Input: part model. Units: mm. Frame: model coordinates. A direction names the side the tool comes from. Coordinates: 2 decimals unless noted, no trailing zeros. Order: outer loops, then holes, each group sorted by start corner. A loop starts at its lowest first (then second) coordinate and runs counter-clockwise, first axis right, second up. Notation, with made-up numbers: (56.25, 69) -> (112.25, 69) arc R22 cw to (112.25, 106) -> close; hole circle Ø3 at (-1, 27). An arc over 180 degrees is marked (long way). Use CSV: the item, a comma, the result in double quotes. Start each with the question number.
```python
from build123d import *

# Parameters (mm, degrees)
BOX002_W          = 4.2
BOX002_H          = 3
BOX002_DEPTH      = 4
CYLINDER005_R     = 2.1
CYLINDER005_DEPTH = 4
CYLINDER004_R     = 2.1
CYLINDER004_DEPTH = 4
BOX003_W          = 9
BOX003_H          = 3
BOX003_DEPTH      = 4
CYLINDER006_R     = 4.5
CYLINDER006_DEPTH = 4
CYLINDER007_R     = 4.5
CYLINDER007_DEPTH = 4
BOX005_W          = 6
BOX005_H          = 8
BOX005_DEPTH      = 4
CHAMFER002_SIZE   = 2
BOX006_W          = 60
BOX006_H          = 8
BOX006_DEPTH      = 4
CHAMFER_SIZE      = 2
CHAMFER003_SIZE   = 2
BOX004_W          = 6
BOX004_H          = 8
BOX004_DEPTH      = 4
CHAMFER001_SIZE   = 2
BOX_W             = 4.2
BOX_H             = 3
BOX_DEPTH         = 4
CYLINDER001_R     = 2.1
CYLINDER001_DEPTH = 4
CYLINDER_R        = 2.1
CYLINDER_DEPTH    = 4
BOX001_W          = 9
BOX001_H          = 3
BOX001_DEPTH      = 4
CYLINDER003_R     = 4.5
CYLINDER003_DEPTH = 4
CYLINDER002_R     = 4.5
CYLINDER002_DEPTH = 4


with BuildPart() as obj1:
    # Box002 → Box002 (new body)
    with BuildSketch(Plane(origin=(-2.1, 0, 0), x_dir=(1, 0, 0), z_dir=(0, 0, 1))):
        with Locations((2.1, 1.5)):
            Rectangle(BOX002_W, BOX002_H)
    extrude(amount=BOX002_DEPTH)


with BuildPart() as zylinder005:
    # Cylinder005 → Cylinder005 (new body)
    with BuildSketch(Plane(origin=(0, 3, 0), x_dir=(1, 0, 0), z_dir=(0, 0, 1))):
        Circle(CYLINDER005_R)
    extrude(amount=CYLINDER005_DEPTH)


with BuildPart() as fusion002:
    # Cylinder004 → Cylinder004 (new body)
    with BuildSketch(Plane.XY):
        Circle(CYLINDER004_R)
    extrude(amount=CYLINDER004_DEPTH)

    # Fusion002: union obj1, Zylinder005
    add(obj1.part)
    add(zylinder005.part)


with BuildPart() as obj2:
    # Box003 → Box003 (new body)
    with BuildSketch(Plane(origin=(-4.5, 0, 0), x_dir=(1, 0, 0), z_dir=(0, 0, 1))):
        with Locations((4.5, 1.5)):
            Rectangle(BOX003_W, BOX003_H)
    extrude(amount=BOX003_DEPTH)


with BuildPart() as zylinder006:
    # Cylinder006 → Cylinder006 (new body)
    with BuildSketch(Plane(origin=(0, 3, 0), x_dir=(1, 0, 0), z_dir=(0, 0, 1))):
        Circle(CYLINDER006_R)
    extrude(amount=CYLINDER006_DEPTH)


with BuildPart() as cut001:
    # Cylinder007 → Cylinder007 (new body)
    with BuildSketch(Plane.XY):
        Circle(CYLINDER007_R)
    extrude(amount=CYLINDER007_DEPTH)

    # Fusion003: union obj2, Zylinder006
    add(obj2.part)
    add(zylinder006.part)

    # Cut001: cut Fusion002
    add(fusion002.part, mode=Mode.SUBTRACT)


with BuildPart() as cut001_1:
    # Cut001 placement: moved
    add(cut001.part.moved(Location((77.5, 0, 0))))


with BuildPart() as chamfer002:
    # Box005 → Box005 (new body)
    with BuildSketch(Plane(origin=(69, -3.5, 0), x_dir=(1, 0, 0), z_dir=(0, 0, 1))):
        with Locations((3, 4)):
            Rectangle(BOX005_W, BOX005_H)
    extrude(amount=BOX005_DEPTH)

    # Chamfer002
    chamfer002_edges = [chamfer002.edges().sort_by_distance(p)[0] for p in [
        (69, 0.5, 0),
    ]]
    chamfer(chamfer002_edges, length=CHAMFER002_SIZE)


with BuildPart() as chamfer003:
    # Box006 → Box006 (new body)
    with BuildSketch(Plane(origin=(11, -3.5, 2), x_dir=(1, 0, 0), z_dir=(0, 0, 1))):
        with Locations((30, 4)):
            Rectangle(BOX006_W, BOX006_H)
    extrude(amount=BOX006_DEPTH)

    # Chamfer
    chamfer_edges = [chamfer003.edges().sort_by_distance(p)[0] for p in [
        (11, 0.5, 6),
    ]]
    chamfer(chamfer_edges, length=CHAMFER_SIZE)

    # Chamfer003
    chamfer003_edges = [chamfer003.edges().sort_by_distance(p)[0] for p in [
        (71, 0.5, 6),
    ]]
    chamfer(chamfer003_edges, length=CHAMFER003_SIZE)


with BuildPart() as fusion004:
    # Box004 → Box004 (new body)
    with BuildSketch(Plane(origin=(7, -3.5, 0), x_dir=(1, 0, 0), z_dir=(0, 0, 1))):
        with Locations((3, 4)):
            Rectangle(BOX004_W, BOX004_H)
    extrude(amount=BOX004_DEPTH)

    # Chamfer001
    chamfer001_edges = [fusion004.edges().sort_by_distance(p)[0] for p in [
        (13, 0.5, 0),
    ]]
    chamfer(chamfer001_edges, length=CHAMFER001_SIZE)

    # Fusion004: union Chamfer002, Chamfer003
    add(chamfer002.part)
    add(chamfer003.part)


with BuildPart() as obj3:
    # Box → Box (new body)
    with BuildSketch(Plane(origin=(-2.1, 0, 0), x_dir=(1, 0, 0), z_dir=(0, 0, 1))):
        with Locations((2.1, 1.5)):
            Rectangle(BOX_W, BOX_H)
    extrude(amount=BOX_DEPTH)


with BuildPart() as zylinder001:
    # Cylinder001 → Cylinder001 (new body)
    with BuildSketch(Plane(origin=(0, 3, 0), x_dir=(1, 0, 0), z_dir=(0, 0, 1))):
        Circle(CYLINDER001_R)
    extrude(amount=CYLINDER001_DEPTH)


with BuildPart() as fusion:
    # Cylinder → Cylinder (new body)
    with BuildSketch(Plane.XY):
        Circle(CYLINDER_R)
    extrude(amount=CYLINDER_DEPTH)

    # Fusion: union obj3, Zylinder001
    add(obj3.part)
    add(zylinder001.part)


with BuildPart() as obj4:
    # Box001 → Box001 (new body)
    with BuildSketch(Plane(origin=(-4.5, 0, 0), x_dir=(1, 0, 0), z_dir=(0, 0, 1))):
        with Locations((4.5, 1.5)):
            Rectangle(BOX001_W, BOX001_H)
    extrude(amount=BOX001_DEPTH)


with BuildPart() as zylinder003:
    # Cylinder003 → Cylinder003 (new body)
    with BuildSketch(Plane(origin=(0, 3, 0), x_dir=(1, 0, 0), z_dir=(0, 0, 1))):
        Circle(CYLINDER003_R)
    extrude(amount=CYLINDER003_DEPTH)


with BuildPart() as fusion005:
    # Cylinder002 → Cylinder002 (new body)
    with BuildSketch(Plane.XY):
        Circle(CYLINDER002_R)
    extrude(amount=CYLINDER002_DEPTH)

    # Fusion001: union obj4, Zylinder003
    add(obj4.part)
    add(zylinder003.part)

    # Cut: cut Fusion
    add(fusion.part, mode=Mode.SUBTRACT)


with BuildPart() as fusion005_1:
    # Cut placement: moved
    add(fusion005.part.moved(Location((4.5, 0, 0))))

    # Fusion005: union Cut001, Fusion004
    add(cut001_1.part)
    add(fusion004.part)


solid = fusion005_1.part
```
1. Pull-direction query (X, two-part tool) for faces 1 (the face through (6.6, 1, 2)), 2 (the face through (12, 0, 5)), 3 (the face through (41, 1, 6)), 4 (the face through (75.4, 1, 2)); classes: released by +X, released by -X, zero draft, split by the parting line, or undercut.
2. Contact query for flat-ended pins moving along their axis: P1, Ø4, axis at x = 52.5, y = 0, coming from the -Z side; P2, Ø2, axis at x = 69.5, z = 4, coming from the -Y side; P3, Ø3, axis at x = 35, z = 3, coming from the +Y side. Output: stop coordinate, or through.
3. Section C-C on y = 1. Return loops of the section in (x, z).
4. Section D-D on z = 5.05. Return loops of the section in (x, y).
5. Section A-A on z = 1. Return loops of the section in (x, y).
6. Section B-B on x = 4.5. Return loops of the section in (y, z).
7. Access query for faces 5 (the face through (41, 4.5, 4)), 6 (the face through (12, 0, 1)), 7 (the face through (7, 2, 4)), 8 (the face through (75, 2, 4)), 9 (the face through (77.5, 5.1, 2)). Directions: +Z, -Z, +X, -X, +Y, -Y. A direction counts if a zero-diameter tool reaches every point of the face in a straight line with its end or side. Return the directions, or none.
8. Material intervals for line 1 along X through (y, z) = (3, 2.15); line 2 along Y through (x, z) = (36, 5); line 3 along Z through (x, y) = (52, 1.25), sorted ascending.
Values follow:
1,face 1,"undercut"
1,face 2,"released by -X"
1,face 3,"zero draft"
1,face 4,"undercut"
2,P1,"stops at z = 2"
2,P2,"stops at y = -3.5"
2,P3,"stops at y = 4.5"
3,outline,"(0, 0) -> (2.4, 0) -> (2.4, 4) -> (0, 4) -> close; (6.6, 0) -> (11, 0) -> (13, 2) -> (69, 2) -> (71, 0) -> (75.4, 0) -> (75.4, 4) -> (71, 4) -> (69, 6) -> (13, 6) -> (11, 4) -> (6.6, 4) -> close; (79.6, 0) -> (82, 0) -> (82, 4) -> (79.6, 4) -> close"
4,outline,"(12.05, -3.5) -> (69.95, -3.5) -> (69.95, 4.5) -> (12.05, 4.5) -> close"
5,outline,"(0, 0) arc R4.5 ccw to (7.33, -3.5) -> (12, -3.5) -> (12, 4.5) -> (8.74, 4.5) arc R4.5 ccw to (0, 3) -> close; (70, -3.5) -> (74.67, -3.5) arc R4.5 ccw to (82, 0) -> (82, 3) arc R4.5 ccw to (73.26, 4.5) -> (70, 4.5) -> close; hole (2.4, 0) arc R2.1 ccw to (6.6, 0) -> (6.6, 3) arc R2.1 ccw to (2.4, 3) -> close; hole (75.4, 0) arc R2.1 ccw to (79.6, 0) -> (79.6, 3) arc R2.1 ccw to (75.4, 3) -> close"
6,outline,"(-4.5, 0) -> (-2.1, 0) -> (-2.1, 4) -> (-4.5, 4) -> close; (5.1, 0) -> (7.5, 0) -> (7.5, 4) -> (5.1, 4) -> close"
7,face 5,"+Z, -Z, +Y"
7,face 6,"-Z, +Y, -Y"
7,face 7,"+Z, -X, +Y, -Y"
7,face 8,"+Z, +X, +Y, -Y"
7,face 9,"+Z, -Z"
8,line 1,"x = 0 to 2.4, 6.6 to 75.4, 79.6 to 82"
8,line 2,"y = -3.5 to 4.5"
8,line 3,"z = 2 to 6"
